Source: CAD feature listing. Evaluate the final solid. Frame: model axes, mm. Face numbers are marked on the shaded views. A direction names the side the tool comes from. Give positions to 0.01 mm unless a question says otherwise; leave off trailing zeros. Order: outer loops, then holes, each group sorted by start corner. A loop starts at its lowest first (then second) coordinate and runs counter-clockwise, first axis right, second up. Notation, with made-up numbers: M 66,35 L 82,35 A30 ccw 82,64 Z; hole C 60,83.25 d5. An arc over 180 degrees is marked long. Answer as a JSON object with one key per item and string values. Group by question number.
1. Pin query (flat end, axial travel): P1, Ø1, axis at x = 11, z = 5.5, coming from the -Y side; P2, Ø0.6, axis at y = -46.5, z = 17.5, coming from the +X side; P3, Ø1, axis at y = -47.5, z = 20, coming from the -X side; P4, Ø2.5, axis at x = -36, y = -46, coming from the +Z side. Return the tip coordinate at first contact, or that it passes through.
2. Section query B-B (y = 46). Output: boundary loops of the cut face in (x, z), plus the area to 3 significant figures.
3. Set-up query: the marked faces 1, 2, 3 and 4. Return all of +Z, -Z, +X, -X, +Y, -Y with unobstructed straight access to the full face (end or side cutting, diameter ignored); none if empty.
4. Section query D-D (z = 8.25). Output: boundary loops of the cut face in (x, y), plus the area to 3 significant figures.
5. Material intervals for L1, parallel to Y at x = 20, z = 2.25; L2, parallel to Y at x = -36, z = 1.3; L3, parallel to Y at x = -46, z = 2.3, sorted ascending. Write a range as [from, to].
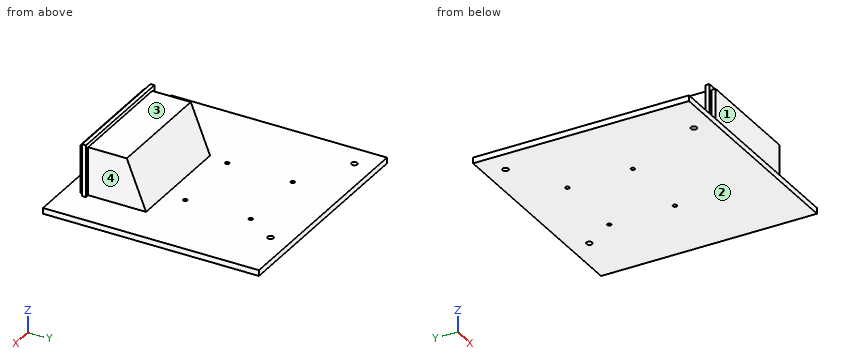
from build123d import *

# Parameters (mm, degrees)
SKETCH1_W           = 116
SKETCH1_H           = 112
BOSS_EXTRUDE1_DEPTH = 3
SKETCH2_W           = 58
SKETCH2_H           = 34
BOSS_EXTRUDE2_DEPTH = 25
CHAMFER1_SIZE2      = 10
CHAMFER1_SIZE       = 25
BOSS_EXTRUDE4_DEPTH = 2
CUT_EXTRUDE1_REACH  = 87.024
SKETCH5_R           = 1.5
CUT_EXTRUDE2_REACH  = 87.024
SKETCH6_R           = 1


with BuildPart() as part:
    # Sketch1 → Boss-Extrude1 (new body)
    with BuildSketch(Plane.XY):
        Rectangle(SKETCH1_W, SKETCH1_H)
    extrude(amount=BOSS_EXTRUDE1_DEPTH)

    # Sketch2 → Boss-Extrude2 (add)
    with BuildSketch(Plane.XY.offset(3)):
        with Locations((9, -31)):
            Rectangle(SKETCH2_W, SKETCH2_H)
    extrude(amount=BOSS_EXTRUDE2_DEPTH)

    # Chamfer1
    chamfer1_edges = [part.edges().sort_by_distance(p)[0] for p in [
        (9, -14, 28),
    ]]
    chamfer1_side = [part.faces().sort_by_distance(p)[0] for p in [
        (9, -14, 27.8),
    ]]
    chamfer(chamfer1_edges, length=CHAMFER1_SIZE - 0.0001, length2=CHAMFER1_SIZE2 - 0.0001, reference=chamfer1_side[0])  # a hair under: the kernel refuses the full size

    # Sketch4 → Boss-Extrude4 (add)
    with BuildSketch(Plane(origin=(0, -46, 0), x_dir=(-1, 0, 0), z_dir=(0, -1, 0))):
        Polygon((22, -3), (20, -3), (20, -28), (-38, -28), (-38, -3), (-40, -3), (-40, -30), (22, -30), align=None)
    extrude(amount=-BOSS_EXTRUDE4_DEPTH)

    # Sketch5 → Cut-Extrude1 (cut, up to next)
    with BuildSketch(Plane.XY.offset(3), mode=Mode.PRIVATE) as cut_extrude1_sk1:
        with Locations((-46, 46)):
            Circle(SKETCH5_R)
    cut_extrude1_tool1 = extrude(cut_extrude1_sk1.sketch, amount=-CUT_EXTRUDE1_REACH, mode=Mode.PRIVATE) & part.part
    # Sketch5 → Cut-Extrude1 (cut, up to next)
    with BuildSketch(Plane.XY.offset(3), mode=Mode.PRIVATE) as cut_extrude1_sk2:
        with Locations((30, 46)):
            Circle(SKETCH5_R)
    cut_extrude1_tool2 = extrude(cut_extrude1_sk2.sketch, amount=-CUT_EXTRUDE1_REACH, mode=Mode.PRIVATE) & part.part
    # Sketch5 → Cut-Extrude1 (cut, up to next)
    with BuildSketch(Plane.XY.offset(3), mode=Mode.PRIVATE) as cut_extrude1_sk3:
        with Locations((-36, -46)):
            Circle(SKETCH5_R)
    cut_extrude1_tool3 = extrude(cut_extrude1_sk3.sketch, amount=-CUT_EXTRUDE1_REACH, mode=Mode.PRIVATE) & part.part
    add(cut_extrude1_tool1.solids().sort_by_distance((-46, 46, 3))[0], mode=Mode.SUBTRACT)
    add(cut_extrude1_tool2.solids().sort_by_distance((30, 46, 3))[0], mode=Mode.SUBTRACT)
    add(cut_extrude1_tool3.solids().sort_by_distance((-36, -46, 3))[0], mode=Mode.SUBTRACT)

    # Sketch6 → Cut-Extrude2 (cut, up to next)
    with BuildSketch(Plane.XY.offset(3), mode=Mode.PRIVATE) as cut_extrude2_sk1:
        with Locations((-18, 30)):
            Circle(SKETCH6_R)
    cut_extrude2_tool1 = extrude(cut_extrude2_sk1.sketch, amount=-CUT_EXTRUDE2_REACH, mode=Mode.PRIVATE) & part.part
    # Sketch6 → Cut-Extrude2 (cut, up to next)
    with BuildSketch(Plane.XY.offset(3), mode=Mode.PRIVATE) as cut_extrude2_sk2:
        with Locations((20, 30)):
            Circle(SKETCH6_R)
    cut_extrude2_tool2 = extrude(cut_extrude2_sk2.sketch, amount=-CUT_EXTRUDE2_REACH, mode=Mode.PRIVATE) & part.part
    # Sketch6 → Cut-Extrude2 (cut, up to next)
    with BuildSketch(Plane.XY.offset(3), mode=Mode.PRIVATE) as cut_extrude2_sk3:
        with Locations((-18, -4)):
            Circle(SKETCH6_R)
    cut_extrude2_tool3 = extrude(cut_extrude2_sk3.sketch, amount=-CUT_EXTRUDE2_REACH, mode=Mode.PRIVATE) & part.part
    # Sketch6 → Cut-Extrude2 (cut, up to next)
    with BuildSketch(Plane.XY.offset(3), mode=Mode.PRIVATE) as cut_extrude2_sk4:
        with Locations((20, -4)):
            Circle(SKETCH6_R)
    cut_extrude2_tool4 = extrude(cut_extrude2_sk4.sketch, amount=-CUT_EXTRUDE2_REACH, mode=Mode.PRIVATE) & part.part
    add(cut_extrude2_tool1.solids().sort_by_distance((-18, 30, 3))[0], mode=Mode.SUBTRACT)
    add(cut_extrude2_tool2.solids().sort_by_distance((20, 30, 3))[0], mode=Mode.SUBTRACT)
    add(cut_extrude2_tool3.solids().sort_by_distance((-18, -4, 3))[0], mode=Mode.SUBTRACT)
    add(cut_extrude2_tool4.solids().sort_by_distance((20, -4, 3))[0], mode=Mode.SUBTRACT)


solid = part.part
Answer sheet:
{
 "1": {"P1": "y = -48", "P2": "x = 38", "P3": "x = -20", "P4": "through"},
 "2": {"outline": "M -58,0 L -47.5,0 L -47.5,3 L -58,3 Z; M -44.5,0 L 28.5,0 L 28.5,3 L -44.5,3 Z; M 31.5,0 L 58,0 L 58,3 L 31.5,3 Z", "area": "330 mm^2"},
 "3": {"face 1": "+Z, +X, -X, -Y", "face 2": "-Z, +X, -X, +Y, -Y", "face 3": "+Z, +X, -X, +Y", "face 4": "+Z, +X, +Y"},
 "4": {"outline": "M -22,-46 L -20,-46 L -20,-48 L 38,-48 L 38,-46 L 40,-46 L 40,-44 L 38,-44 L 38,-16.1 L -20,-16.1 L -20,-44 L -22,-44 Z", "area": "1,860 mm^2"},
 "5": {"L1": "[-56, -5], [-3, 29], [31, 56]", "L2": "[-56, -47.5], [-44.5, 56]", "L3": "[-56, 44.5], [47.5, 56]"}
}
